Design review of the part built by this model. Coordinates are the model's own, in mm. Coordinates: 2 decimals unless noted, no trailing zeros. Write each loop counter-clockwise with the first axis right and the second up, starting at its lowest first coordinate (ties: lowest second). Pieces come first, ordered by that corner, then holes. Notation, with made-up numbers: (-18, -39.75) - (28, -39.75) arc R15 ccw to (28, -23.75) - close; hole circle Ø2 at (42.5, 3). An arc over 180 degrees is marked (long way). Answer as a JSON object with one key per item and string values.
```python
from build123d import *

# Parameters (mm, degrees)
SKETCH3_R           = 13.25
BOSS_EXTRUDE1_DEPTH = 6.35
SKETCH4_R           = 5
SKETCH4_R_2         = 1.25
CUT_EXTRUDE1_DEPTH  = 6.35


with BuildPart() as part:
    # Sketch3 → Boss-Extrude1 (new body)
    with BuildSketch(Plane.XY):
        Circle(SKETCH3_R)
    extrude(amount=BOSS_EXTRUDE1_DEPTH)

    # Sketch4 → Cut-Extrude1 (cut)
    with BuildSketch(Plane.XY.offset(6.35)):
        Circle(SKETCH4_R)
        with Locations((0, 9.75)):
            Circle(SKETCH4_R_2)
        with Locations((9.75, 0)):
            Circle(SKETCH4_R_2)
        with Locations((0, -9.75)):
            Circle(SKETCH4_R_2)
        with Locations((-9.75, 0)):
            Circle(SKETCH4_R_2)
    extrude(amount=-CUT_EXTRUDE1_DEPTH, mode=Mode.SUBTRACT)


solid = part.part
```
(1) The part is to be moulded in two halves that separate along Y. For faces 1 (the face through (-1.08, -4.88, 3.22)), 2 (the face through (7.123, 11.172, 3.131)), 3 (the face through (6, 0, 6.35)), say which applies: pulls with the +Y half, pulls with the -Y half, needs draft (parallel to the pull), parting line crosses it, or undercut.
Solved:
{"face 1": "undercut", "face 2": "parting line crosses it", "face 3": "needs draft"}
(2) For pin 1 (3 mm diameter, centred on x = -9.75, y = 0, fed in from -Z); pin 2 (4 mm diameter, centred on x = -0.5, y = -2, fed in from -Z); pin 3 (2 mm diameter, centred on x = -4.5, z = 4.5, fed in from +Y); pin 4 (1.5 mm diameter, centred on y = -7.5, z = 4.5, fed in from +X), all flat-tipped, find the tip position at first contact; note any pin that passes through.
Solved:
{"pin 1": "stops at z = 0", "pin 2": "passes through", "pin 3": "stops at y = 12.78", "pin 4": "stops at x = 11.4"}
(3) To check wall thickness, follow line 1 (Y direction, x = 0, z = 4.75); line 2 (Y direction, x = -10.5, z = 3.75); line 3 (X direction, y = 4.5, z = 3.5). State the ranges of each line that lie inside material, in increasing order. Write a range as from..to.
Solved:
{"line 1": "y = -13.25..-11, -8.5..-5, 5..8.5, 11..13.25", "line 2": "y = -8.08..-1, 1..8.08", "line 3": "x = -12.46..-2.18, 2.18..12.46"}
(4) Take a section at D-D, the plane y = -10.5. Write out the cut boundary in (x, z), and give its area (3 significant figures).
Solved:
{"outline": "(-8.08, 0) - (-1, 0) - (-1, 6.35) - (-8.08, 6.35) - close; (1, 0) - (8.08, 0) - (8.08, 6.35) - (1, 6.35) - close", "area": "89.9 mm^2"}
(5) Take a section at A-A, the plane x = 0. Write out the cut boundary in (y, z), and give its area (3 significant figures).
Solved:
{"outline": "(-13.25, 0) - (-11, 0) - (-11, 6.35) - (-13.25, 6.35) - close; (-8.5, 0) - (-5, 0) - (-5, 6.35) - (-8.5, 6.35) - close; (5, 0) - (8.5, 0) - (8.5, 6.35) - (5, 6.35) - close; (11, 0) - (13.25, 0) - (13.25, 6.35) - (11, 6.35) - close", "area": "73.0 mm^2"}
(6) Take a section at C-C, the plane z = 3.75. Write out the cut boundary in (x, y), and give its area (3 significant figures).
Solved:
{"outline": "circle Ø26.5 at (0, 0); hole circle Ø2.5 at (-9.75, 0); hole circle Ø10 at (0, 0); hole circle Ø2.5 at (0, -9.75); hole circle Ø2.5 at (0, 9.75); hole circle Ø2.5 at (9.75, 0)", "area": "453 mm^2"}
